Could you check a few things on this drawing? It's one solid part, dimensions in mm from its lowest x, y, z. Coordinates: 2 decimals unless noted, no trailing zeros. Loops run counter-clockwise (first coordinate to the right, second up) from the corner with the lowest first, then second, coordinate; pieces in that order, holes last. Notation, with made-up numbers: M -21,-12 L 29,-12 A26 ccw 29,15 Z; hole C -21.75,53.25 d5. An arc over 180 degrees is marked long. Answer as a JSON object with one key per item and string values. Group by question number.
Item 1: Suppose I cut it at B-B (y = 2.5). Write out the boundary of the cut face in (x, z), then the cut area to 4 significant figures.
Item 2: We'd pull the mould along X, two halves only. Please class the marked faces 1 and 2: +X half, -X half, draft (parallel to the pull), parting line (faces both ways), or undercut.
Item 3: I'm going to push flat-ended pins straight in: pin 1 Ø15 at (x, z) = (43.5, 49.5) entering from +Y; pin 2 Ø11 at (x, z) = (50, 90) entering from -Y; pin 3 Ø1 at (y, z) = (1, 81) entering from +X. Where does each tip first touch, or does it pass through?
Item 4: If I drill on line 1 (X direction, y = 2, z = 30) (1 decimal); line 2 (X direction, y = 2.6, z = 29) (1 decimal); line 3 (Z direction, x = 17, y = 2.2), over which ranges is the centre line in solid material (lowest first)?
Item 5: Suppose I cut it at A-A (x = 50). Count the separate pieces of the cut face and the enclosed holes in it, then the cut area to 3 significant figures.
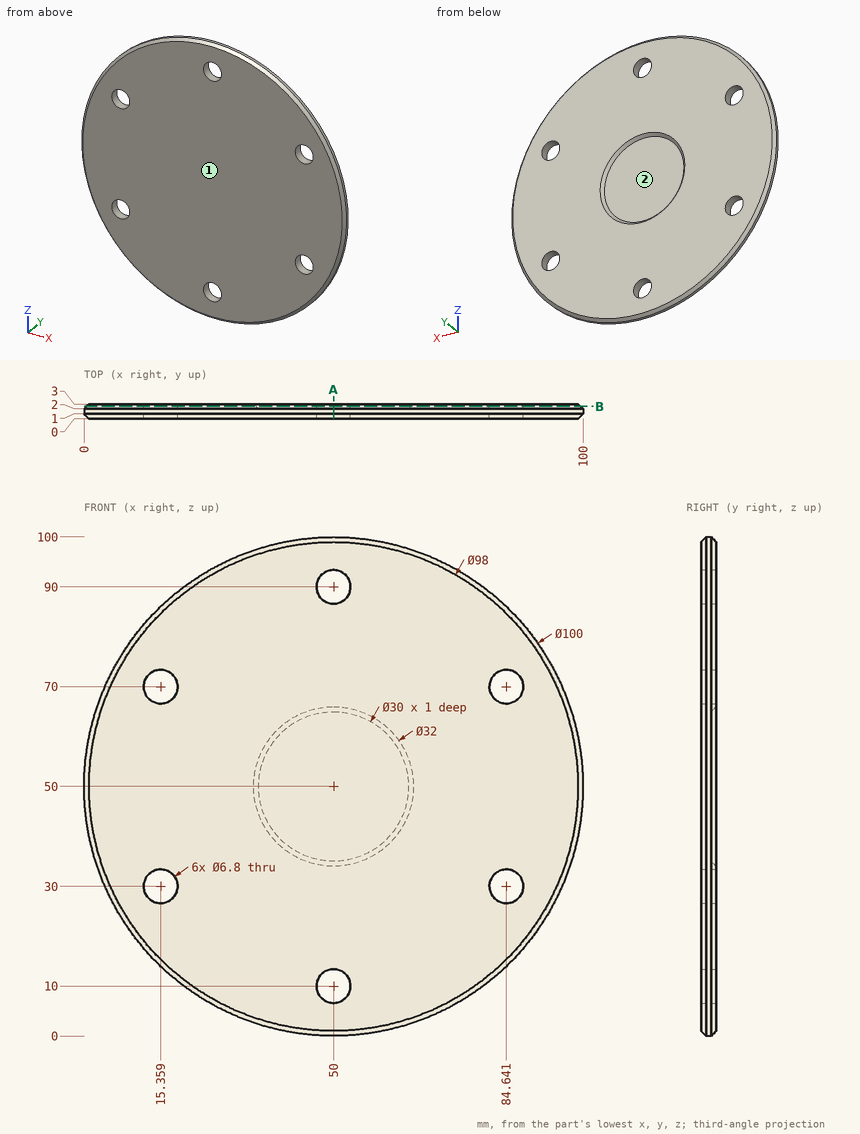
From the geometry:
{
 "1": {"outline": "C 50,50 d99; hole C 15.36,30 d6.8; hole C 15.36,70 d6.8; hole C 50,50 d31; hole C 50,10 d6.8; hole C 50,90 d6.8; hole C 84.64,30 d6.8; hole C 84.64,70 d6.8", "area": "6,725 mm2"},
 "2": {"face 1": "draft", "face 2": "undercut"},
 "3": {"pin 1": "y = 2", "pin 2": "y = 0", "pin 3": "x = 89.62"},
 "4": {"line 1": "4.2 to 12, 18.8 to 81.2, 88 to 95.8", "line 2": "5.3 to 12.1, 18.6 to 81.4, 87.9 to 94.7", "line 3": "12.7 to 27.02, 32.98 to 67.02, 72.98 to 87.3"},
 "5": {"separate pieces": "3", "enclosed holes": "0", "area": "226 mm2"}
}
